For this review, take the finished solid that the model builds, in its own axes (mm). Face numbers are marked on the shaded views. A direction names the side the tool comes from. Give positions to 0.01 mm unless a question says otherwise; leave off trailing zeros. Order: outer loops, then holes, each group sorted by start corner. A loop starts at its lowest first (then second) coordinate and runs counter-clockwise, first axis right, second up. Notation, with made-up numbers: (78, 84.5) - (97, 84.5) arc R12 ccw to (97, 98.5) - close; hole circle Ø5 at (34, 50). An arc over 180 degrees is marked (long way). Answer as a JSON object with one key per item and string values. Group by question number.
from build123d import *
from build123d.topology import SkipClean

# Parameters (mm, degrees)
ESQUISSE2_W             = 35
ESQUISSE2_H             = 35
ESQUISSE2_W_2           = 55
ESQUISSE2_H_2           = 80
BOSS_EXTRU_1_DEPTH      = 38
BOSS_EXTRU_2_START      = -1
BOSS_EXTRU_2_DEPTH      = 1
CONG_2_R                = 4
ESQUISSE3_W             = 55
ESQUISSE3_H             = 17
ENL_V_MAT_EXTRU_1_DEPTH = 195.551407124
ESQUISSE4_W             = 10
ESQUISSE4_H             = 13
ENL_V_MAT_EXTRU_2_DEPTH = 138.841394442
ESQUISSE5_R             = 1.65
BOSS_EXTRU_3_DEPTH      = 1.8
ESQUISSE6_R             = 2.5
BOSS_EXTRU_4_DEPTH      = 2.6
ESQUISSE6_3_R           = 1.25
BOSS_EXTRU_5_DEPTH      = 5


with BuildPart() as part:
    # Esquisse2 → Boss.-Extru.1 (new body)
    with BuildSketch(Plane(origin=(0, 0, 0), x_dir=(1, 0, 0), z_dir=(0, 1, 0))):
        with BuildLine():
            Line((-65.996632911, 23.333333333), (-37.712361663, 103.333333333))
            ThreePointArc((-37.712361663, 103.333333333), (0, 130), (37.712361663, 103.333333333))
            Line((37.712361663, 103.333333333), (65.996632911, 23.333333333))
            ThreePointArc((65.996632911, 23.333333333), (0, -70), (-65.996632911, 23.333333333))
        make_face()
        Rectangle(ESQUISSE2_W, ESQUISSE2_H, mode=Mode.SUBTRACT)
        with Locations((0, 67.5)):
            Rectangle(ESQUISSE2_W_2, ESQUISSE2_H_2, mode=Mode.SUBTRACT)
    extrude(amount=BOSS_EXTRU_1_DEPTH)

    # Esquisse2<2> → Boss.-Extru.2 (add)
    with SkipClean():  # the faces are left unmerged after this step: merging them gives an invalid solid
        with BuildSketch(Plane(origin=(0, 0, 0), x_dir=(1, 0, 0), z_dir=(0, 1, 0)).offset(BOSS_EXTRU_2_START)):
            with BuildLine():
                Line((-37.712361663, 103.333333333), (-65.996632911, 23.333333333))
                ThreePointArc((-65.996632911, 23.333333333), (0, -70), (65.996632911, 23.333333333))
                Line((65.996632911, 23.333333333), (37.712361663, 103.333333333))
                ThreePointArc((37.712361663, 103.333333333), (0, 130), (-37.712361663, 103.333333333))
            make_face()
        extrude(amount=BOSS_EXTRU_2_DEPTH)

    # Congé2
    # the kernel refuses this fillet: 4 mm, written as the material it takes off along each edge
    with BuildSketch(Plane(origin=(0, -1, 0), x_dir=(-0.9428090415820636, 0, -0.33333333333333304), z_dir=(0.33333333333333304, 0, -0.9428090415820636))) as cong_2_piece_1:
        with BuildLine():
            CenterArc((70 - CONG_2_R, CONG_2_R), CONG_2_R, 270, 90)
            Line((70 - CONG_2_R, 0), (70, 0))
            Line((70, 0), (70, CONG_2_R))
        make_face()
    revolve(axis=Axis((0, -1, 0), (0, 1, 0)), revolution_arc=218.942441269, mode=Mode.SUBTRACT)
    with BuildSketch(Plane(origin=(65.996632911, -1, -23.333333333), x_dir=(-0.9428090415820634, 0, 0.33333333333333354), z_dir=(-0.33333333333333354, 0, -0.9428090415820634))) as cong_2_piece_2:
        with BuildLine():
            CenterArc((CONG_2_R, CONG_2_R), CONG_2_R, 180, 90)
            Line((0, CONG_2_R), (0, 0))
            Line((0, 0), (CONG_2_R, 0))
        make_face()
    extrude(amount=84.852813742, mode=Mode.SUBTRACT)
    with BuildSketch(Plane(origin=(-37.712361663, -1, -103.333333333), x_dir=(0, 1, 0), z_dir=(-0.3333333333333333, 0, 0.9428090415820635))) as cong_2_piece_3:
        with BuildLine():
            CenterArc((CONG_2_R, -CONG_2_R), CONG_2_R, 90, 90)
            Line((0, -CONG_2_R), (0, 0))
            Line((0, 0), (CONG_2_R, 0))
        make_face()
    extrude(amount=84.852813742, mode=Mode.SUBTRACT)
    with BuildSketch(Plane(origin=(0, -1, -90), x_dir=(0.9428090415820632, 0, -0.3333333333333337), z_dir=(0.3333333333333337, 0, 0.9428090415820632))) as cong_2_piece_4:
        with BuildLine():
            CenterArc((40 - CONG_2_R, CONG_2_R), CONG_2_R, 270, 90)
            Line((40 - CONG_2_R, 0), (40, 0))
            Line((40, 0), (40, CONG_2_R))
        make_face()
    revolve(axis=Axis((0, -1, -90), (0, 1, 0)), revolution_arc=141.057558731, mode=Mode.SUBTRACT)

    # Esquisse3 → Enlèv. mat.-Extru.1 (cut, through all)
    with BuildSketch(Plane.XY.offset(-107.5)):
        with Locations((0, 8.5)):
            Rectangle(ESQUISSE3_W, ESQUISSE3_H)
    extrude(amount=-ENL_V_MAT_EXTRU_1_DEPTH, mode=Mode.SUBTRACT)

    # Esquisse4 → Enlèv. mat.-Extru.2 (cut, through all)
    with BuildSketch(Plane.XY.offset(-17.5)):
        with Locations((0, 6.5)):
            Rectangle(ESQUISSE4_W, ESQUISSE4_H)
    extrude(amount=-ENL_V_MAT_EXTRU_2_DEPTH, mode=Mode.SUBTRACT)

    # Esquisse5 → Boss.-Extru.3 (add)
    # profile 1 of 2: a face of its own
    with BuildSketch(Plane(origin=(0, 38, 0), x_dir=(1, 0, 0), z_dir=(0, 1, 0))):
        with BuildLine():
            Line((-9.5, -17.5), (-9.5, -13))
            ThreePointArc((-9.5, -13), (-10.525126266, -10.525126266), (-13, -9.5))
            Line((-13, -9.5), (-17.5, -9.5))
            Line((-17.5, -9.5), (-17.5, -17.5))
            Line((-17.5, -17.5), (-9.5, -17.5))
        make_face()
        with Locations(Location((-13, -13, 0), (0, 0, 270))):
            Circle(ESQUISSE5_R, mode=Mode.SUBTRACT)
    # profile 2 of 2: a face of its own
    with BuildSketch(Plane(origin=(0, 38, 0), x_dir=(1, 0, 0), z_dir=(0, 1, 0))):
        with BuildLine():
            Line((13, 9.5), (17.5, 9.5))
            Line((17.5, 9.5), (17.5, 17.5))
            Line((17.5, 17.5), (9.5, 17.5))
            Line((9.5, 17.5), (9.5, 13))
            ThreePointArc((9.5, 13), (10.525126266, 10.525126266), (13, 9.5))
        make_face()
        with Locations(Location((13, 13, 0), (0, 0, 270))):
            Circle(ESQUISSE5_R, mode=Mode.SUBTRACT)
    extrude(amount=-BOSS_EXTRU_3_DEPTH)

    # Esquisse6 → Boss.-Extru.4 (add)
    with BuildSketch(Plane(origin=(0, 0, 0), x_dir=(1, 0, 0), z_dir=(0, 1, 0))):
        with Locations(Location((-24.0300102, 87.0767006, 0), (0, 0, 90))):
            Circle(ESQUISSE6_R)
    extrude(amount=BOSS_EXTRU_4_DEPTH)

    # Esquisse6<3> → Boss.-Extru.5 (add)
    with BuildSketch(Plane(origin=(0, 0, 0), x_dir=(1, 0, 0), z_dir=(0, 1, 0))):
        with Locations(Location((-18.9500102, 35.0067006, 0), (0, 0, 270))):
            Circle(ESQUISSE6_3_R)
        with Locations(Location((8.9899898, 35.0067006, 0), (0, 0, 270))):
            Circle(ESQUISSE6_3_R)
        with Locations(Location((24.2299898, 85.8067006, 0), (0, 0, 270))):
            Circle(ESQUISSE6_3_R)
        with Locations(Location((-24.0300102, 87.0767006, 0), (0, 0, 270))):
            Circle(ESQUISSE6_3_R)
    extrude(amount=BOSS_EXTRU_5_DEPTH)


solid = part.part
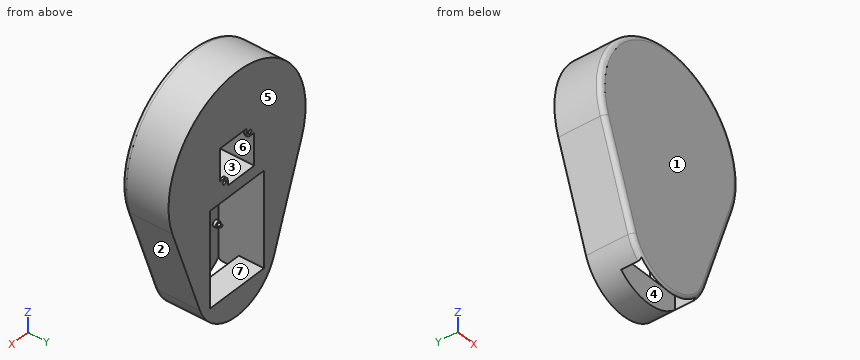
1) Consider section C-C (z = 0). Give the boundary of the cut face in (x, y).
2) For line 1 (Z direction, x = 1, y = 33); line 2 (Y direction, x = -3.5, z = -114.5); line 3 (Y direction, x = -3.5, z = -100), list the stretches that pass through material, from the lowest coordinate up.
3) For pin 1 (5 mm diameter, centred on x = 32.5, y = 27.5, fed in from +Z); pin 2 (2 mm diameter, centred on x = -4.5, z = -78, fed in from +Y); pin 3 (0.9 mm diameter, centred on y = 37, z = -16, fed in from -X), all flat-tipped, find the tip position at first contact; note any pin that passes through.
4) Consider section B-B (y = 29). Give the boundary of the cut face in (x, z), plus the area to 3 significant figures.
5) For the marked faces 4, 5, 6 and 7, list the 3-axis set-ups (+Z, -Z, +X, -X, +Y, -Y) from which the entire face can be reached by the end or side of a thin tool; tool diameter is ignored.
6) Mouldability with a two-part tool opening along Z and no side actions: class the marked faces 1, 2 and 3 as released by +Z, released by -Z, zero draft, split by the parting line, or undercut.
7) Consider section A-A (x = 0). Give the boundary of the cut face in (y, z).
Result set:
{
 "1": {"outline": "(-70, 3) arc R4 ccw to (-66, -1) - (66, -1) arc R4 ccw to (70, 3) - (70, 38) - (17.5, 38) - (17.5, 0) - (-17.5, 0) - (-17.5, 38) - (-70, 38) - close"},
 "2": {"line 1": "z = -129.99 to -107.5, -27.5 to -17.5, 17.5 to 69.99", "line 2": "y = -1 to 0, 17 to 38", "line 3": "y = -1 to 0"},
 "3": {"pin 1": "stops at z = 63.25", "pin 2": "stops at y = 0", "pin 3": "stops at x = -68.25"},
 "4": {"outline": "(-66, -23.33) - (-37.71, -103.33) arc R40 ccw to (37.71, -103.33) - (66, -23.33) arc R70 ccw (long way) to start; hole (-27.5, -107.5) - (27.5, -107.5) - (27.5, -27.5) - (-27.5, -27.5) - close; hole (-17.5, -17.5) - (17.5, -17.5) - (17.5, 17.5) - (-17.5, 17.5) - close", "area": "15,000 mm2"},
 "5": {"face 4": "-Z", "face 5": "+Z, -Z, +X, -X, +Y", "face 6": "none", "face 7": "+Y"},
 "6": {"face 1": "zero draft", "face 2": "released by -Z", "face 3": "undercut"},
 "7": {"outline": "(-1, -126) arc R4 ccw to (0, -128.65) - (0, 17.5) - (38, 17.5) - (38, 70) - (3, 70) arc R4 ccw to (-1, 66) - close; (13, -27.5) - (38, -27.5) - (38, -17.5) - (13, -17.5) - close; (17, -130) - (38, -130) - (38, -107.5) - (17, -107.5) - close"}
}
